Input: part model. Units: mm. Frame: model coordinates. A direction names the side the tool comes from. Give positions to 0.01 mm unless a question says otherwise; leave off trailing zeros. Loops run counter-clockwise (first coordinate to the right, second up) from the corner with the lowest first, then second, coordinate; pieces in that order, holes last. Notation, with made-up numbers: (29.25, 80.5) -> (86.25, 80.5) arc R17 cw to (86.25, 92.5) -> close; hole circle Ø4 at (67.25, 25.25). An arc over 180 degrees is marked (long way). Answer as a JSON object with one key per item and string values. Group by question number.
```python
from build123d import *

# Parameters (mm, degrees)
F3_DEPTH = 25
F7_DEPTH = 8
F8_DEPTH = 12.7


with BuildPart() as f1:
    # F0 (on Top) → F1 (revolve)
    with BuildSketch(Plane.XY):
        with BuildLine():
            Line((6, 22), (6, 16))
            Line((6, 16), (22.248531, 16))
            Line((22.248531, 16), (22.522323, 16))
            Line((22.522323, 16), (22, 0))
            Line((22, 0), (30, 0))
            ThreePointArc((30, 0), (35.17496, 39.465047), (53.825141, 74.628109))
            ThreePointArc((53.825141, 74.628109), (53.428757, 77.857858), (50.763307, 79.724346))
            Line((50.763307, 79.724346), (48, 79.724346))
            Line((48, 79.724346), (48, 87.724346))
            Line((48, 87.724346), (40, 87.724346))
            Line((40, 87.724346), (40, 80))
            Line((40, 80), (40, 68.826427))
            ThreePointArc((40, 68.826427), (39.137165, 67.419082), (38.293772, 66))
            ThreePointArc((38.293772, 66), (28.503213, 44.747977), (23.022968, 22))
            Line((23.022968, 22), (6, 22))
        make_face()
    revolve(axis=Axis((0, 86, 0), (0, 1, 0)))

    # F2 (on face) → F3 (cut)
    with BuildSketch(Plane.XZ.offset(-16)):
        with BuildLine():
            ThreePointArc((3, 14), (-0.160946, 16.99568), (-2.982731, 13.678571))
            ThreePointArc((-2.982731, 13.678571), (0, 11), (2.982731, 13.678571))
            ThreePointArc((2.982731, 13.678571), (2.99568, 13.839054), (3, 14))
        make_face()
        with BuildLine():
            ThreePointArc((13.678571, 2.982731), (11, 0), (13.678571, -2.982731))
            ThreePointArc((13.678571, -2.982731), (16.004459, -2.232071), (17, 0))
            ThreePointArc((17, 0), (16.004459, 2.232071), (13.678571, 2.982731))
        make_face()
        with BuildLine():
            ThreePointArc((2.982731, -13.678571), (0, -11), (-2.982731, -13.678571))
            ThreePointArc((-2.982731, -13.678571), (-0.160946, -16.99568), (3, -14))
            ThreePointArc((3, -14), (2.99568, -13.839054), (2.982731, -13.678571))
        make_face()
        with BuildLine():
            ThreePointArc((-13.678571, 2.982731), (-17, 0), (-13.678571, -2.982731))
            ThreePointArc((-13.678571, -2.982731), (-11.767929, -2.004459), (-11, 0))
            ThreePointArc((-11, 0), (-11.767929, 2.004459), (-13.678571, 2.982731))
        make_face()
    extrude(amount=-F3_DEPTH, mode=Mode.SUBTRACT)

    # F6 (on face) → F7 (join)
    with BuildSketch(Plane(origin=(9.919347, -4.033802, 0), x_dir=(0.376703, 0.926334, 0), z_dir=(0.926334, -0.376703, 0))):
        with BuildLine():
            Line((75.603179, -12.171984), (75.603179, 0))
            Line((75.603179, 0), (75.603179, 12.171984))
            ThreePointArc((75.603179, 12.171984), (74.138713, 15.707518), (70.603179, 17.171984))
            Line((70.603179, 17.171984), (61.603179, 17.171984))
            ThreePointArc((61.603179, 17.171984), (58.067646, 15.707518), (56.603179, 12.171984))
            Line((56.603179, 12.171984), (56.603179, 0))
            Line((56.603179, 0), (56.603179, -12.171984))
            ThreePointArc((56.603179, -12.171984), (58.067646, -15.707518), (61.603179, -17.171984))
            Line((61.603179, -17.171984), (70.603179, -17.171984))
            ThreePointArc((70.603179, -17.171984), (74.138713, -15.707518), (75.603179, -12.171984))
        make_face()
        with BuildLine():
            Line((72.603179, 9.171984), (72.603179, 0))
            Line((72.603179, 0), (72.603179, -9.171984))
            ThreePointArc((72.603179, -9.171984), (71.138713, -12.707518), (67.603179, -14.171984))
            Line((67.603179, -14.171984), (64.603179, -14.171984))
            ThreePointArc((64.603179, -14.171984), (61.067646, -12.707518), (59.603179, -9.171984))
            Line((59.603179, -9.171984), (59.603179, 0))
            Line((59.603179, 0), (59.603179, 9.171984))
            ThreePointArc((59.603179, 9.171984), (61.067646, 12.707518), (64.603179, 14.171984))
            Line((64.603179, 14.171984), (67.603179, 14.171984))
            ThreePointArc((67.603179, 14.171984), (71.138713, 12.707518), (72.603179, 9.171984))
        make_face(mode=Mode.SUBTRACT)
    extrude(amount=F7_DEPTH)

    # F6 (on face) → F8 (cut, symmetric)
    with BuildSketch(Plane(origin=(9.919347, -4.033802, 0), x_dir=(0.376703, 0.926334, 0), z_dir=(0.926334, -0.376703, 0))):
        with BuildLine():
            Line((72.603179, -9.171984), (72.603179, 0))
            Line((72.603179, 0), (72.603179, 9.171984))
            ThreePointArc((72.603179, 9.171984), (71.138713, 12.707518), (67.603179, 14.171984))
            Line((67.603179, 14.171984), (64.603179, 14.171984))
            ThreePointArc((64.603179, 14.171984), (61.067646, 12.707518), (59.603179, 9.171984))
            Line((59.603179, 9.171984), (59.603179, 0))
            Line((59.603179, 0), (59.603179, -9.171984))
            ThreePointArc((59.603179, -9.171984), (61.067646, -12.707518), (64.603179, -14.171984))
            Line((64.603179, -14.171984), (67.603179, -14.171984))
            ThreePointArc((67.603179, -14.171984), (71.138713, -12.707518), (72.603179, -9.171984))
        make_face()
    extrude(amount=F8_DEPTH, both=True, mode=Mode.SUBTRACT)


solid = f1.part
```
Q1. Ray query, probe 1 along X at (y, z) = (83, 0); probe 2 along X at (y, z) = (61, -26). Return the intervals inside material, ascending.
Q2. Set-up query: faces 5 (the face through (45, 79.724, 19)), 6 (the face through (40, 55, -17.172)), 7 (the face through (37, 56, -14.172)). Return all of +Z, -Z, +X, -X, +Y, -Y with unobstructed straight access to the full face (end or side cutting, diameter ignored); none if empty.
Q3. Section B-B on y = 82. Return the cut outline in (x, z).
Q4. Pull-direction query (X, two-part tool) for faces 1 (the face through (34.812, 50.186, -0.128)), 2 (the face through (-8.67, 78.14, 39.05)), 3 (the face through (-18, 87.724, -36)), 4 (the face through (5, 22, 5)); classes: +X half, -X half, draft (parallel to the pull), parting line (faces both ways), or undercut.
Q5. Section C-C on y = 30.5. Return the cut outline in (x, z), then the cut area to 3 significant figures.
Q6. Section A-A on x = 0. State how many separate pieces and enclosed holes the cut face has, then the cut area to 3 significant figures.
Q7. Pin query (flat end, axial travel): pin 1 Ø14 at (x, z) = (8.5, -10.5) entering from +Y; pin 2 Ø2.5 at (x, y) = (40, 54.5) entering from +Z; pin 3 Ø3 at (y, z) = (47.5, -12) entering from -X. Return the tip coordinate at first contact, or that it passes through.
Numbers:
{
 "1": {"probe 1": "x = -48 to -40, 40 to 48", "probe 2": "x = -36.29 to -24.21, 24.21 to 36.29"},
 "2": {"face 5": "+Y", "face 6": "-Z, +X, -Y", "face 7": "none"},
 "3": {"outline": "circle Ø96 at (0, 0); hole circle Ø80 at (0, 0)"},
 "4": {"face 1": "+X half", "face 2": "undercut", "face 3": "draft", "face 4": "undercut"},
 "5": {"outline": "circle Ø65.44 at (0, 0); hole circle Ø49.05 at (0, 0)", "area": "1,470 mm²"},
 "6": {"separate pieces": "4", "enclosed holes": "0", "area": "1,680 mm²"},
 "7": {"pin 1": "stops at y = 22", "pin 2": "stops at z = 17.17", "pin 3": "stops at x = -36.95"}
}
